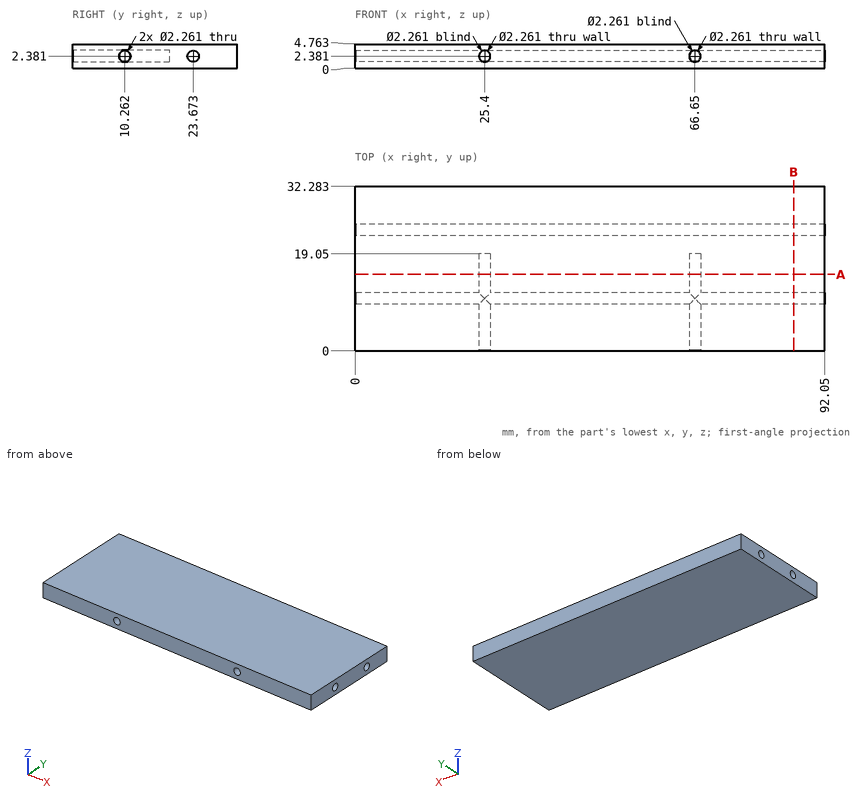
Study the drawing (mm; zero at the part's minimum x, y, z) and answer. Coordinates: 2 decimals unless noted, no trailing zeros. Write each loop counter-clockwise with the first axis right and the second up, starting at its lowest first coordinate (ties: lowest second). Pieces come first, ordered by that corner, then holes. Notation, with made-up numbers: (50.25, -22.75) - (57.25, -22.75) arc R29 cw to (57.25, 16.25) - close; hole circle Ø7 at (-7, 73). An arc over 180 degrees is marked (long way). Answer as a JSON object with one key per item and string values.
Q1. Given pin 1 Ø1.1 at (x, z) = (26, 2) entering from -Y; pin 2 Ø1.1 at (x, z) = (66.5, 2) entering from -Y, each flat-ended and moving along its own axis, determine where each tip first touches the part or whether it passes through.
Results list:
{"pin 1": "stops at y = 0", "pin 2": "stops at y = 19.05"}
Q2. Find section B-B (x = 86). Write down the section's boundary in (y, z).
Results list:
{"outline": "(0, 0) - (32.28, 0) - (32.28, 4.76) - (0, 4.76) - close; hole circle Ø2.26 at (10.26, 2.38); hole circle Ø2.26 at (23.67, 2.38)"}
Q3. Consider L1, parallel to Y at x = 10.5, z = 2.2 (1 decimal); L2, parallel to Y at x = 68, z = 2.8 (1 decimal); L3, parallel to Z at x = 25.4, y = 16.25. Determine where each line is inside the solid, lowest interval first. Write a range as from..to.
Results list:
{"L1": "y = 0..9.1, 11.4..22.6, 24.8..32.3", "L2": "y = 0..9.2, 11.3..22.6, 24.7..32.3", "L3": "z = 0..1.25, 3.51..4.76"}
Q4. Find section A-A (y = 15). Write down the section's boundary in (x, z).
Results list:
{"outline": "(0, 0) - (92.05, 0) - (92.05, 4.76) - (0, 4.76) - close; hole circle Ø2.26 at (25.4, 2.38); hole circle Ø2.26 at (66.65, 2.38)"}
